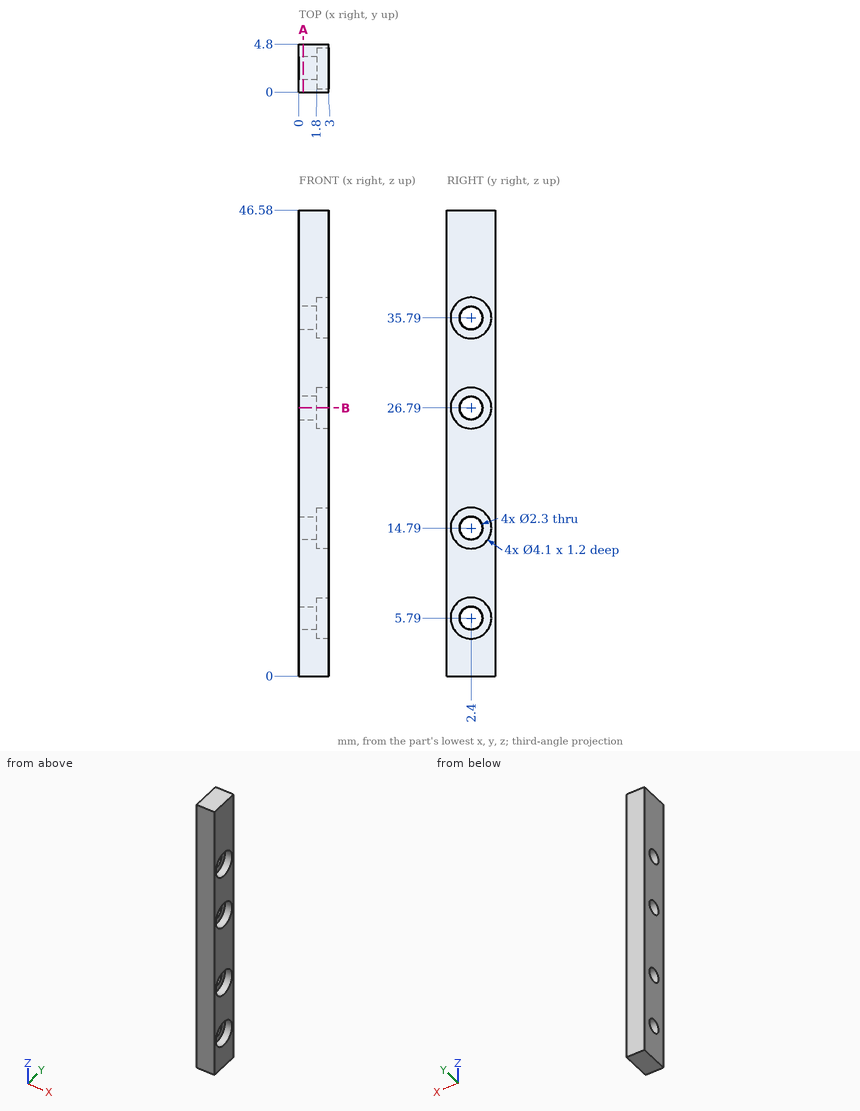
For this review, use the dimensioned drawing (mm, ordinates from the lowest corner) and the shaded views. Round coordinates to 2 decimals unless told otherwise and drop trailing zeros. Write each loop counter-clockwise with the first axis right and the second up, starting at its lowest first coordinate (ties: lowest second). Pieces come first, ordered by that corner, then holes. Notation, with made-up numbers: M 23,-5 L 70,-5 A28 ccw 70,20 Z; hole C 37.5,41 d9. An arc over 180 degrees is marked long. Answer as CSV lines item,"result". Start each with the question number.
Q1. Clearance check with a flat-ended pin moving along its axis: P1, Ø1.2, axis at y = 2.5, z = 35, coming from the +X side. State where the tip first meets the part, or that it passes through.
Q2. Consider section B-B, the plane z = 26.79. Give the boundary of the cut face in (x, y), then the cut area to 3 significant figures.
Q3. Consider section A-A, the plane x = 0.45. Give the boundary of the cut face in (y, z), then the cut area to 3 significant figures.
Q4. Wall thickness on line 1 along Z through (x, y) = (0.6, 2.4); line 2 along Y through (x, z) = (1, 5.79); line 3 along Z through (x, y) = (2.7, 3.8): over which ranges is each line inside the solid? List them lowest first.
Result set:
1,P1,"stops at x = 1.8"
2,outline,"M 0,0 L 3,0 L 3,0.35 L 1.8,0.35 L 1.8,1.25 L 0,1.25 Z; M 0,3.55 L 1.8,3.55 L 1.8,4.45 L 3,4.45 L 3,4.8 L 0,4.8 Z"
2,area,"5.34 mm²"
3,outline,"M 0,0 L 4.8,0 L 4.8,46.58 L 0,46.58 Z; hole C 2.4,5.79 d2.3; hole C 2.4,14.79 d2.3; hole C 2.4,26.79 d2.3; hole C 2.4,35.79 d2.3"
3,area,"207 mm²"
4,line 1,"z = 0 to 4.64, 6.94 to 13.64, 15.94 to 25.64, 27.94 to 34.64, 36.94 to 46.58"
4,line 2,"y = 0 to 1.25, 3.55 to 4.8"
4,line 3,"z = 0 to 4.29, 7.29 to 13.29, 16.29 to 25.29, 28.29 to 34.29, 37.29 to 46.58"
